from build123d import *

# Parameters (mm, degrees)
SKETCH1_W                    = 220
SKETCH1_H                    = 120
BOSS_EXTRUDE1_DEPTH          = 10
CUT_EXTRUDE1_REACH           = 127.698
SKETCH2_W                    = 20.632503002
SKETCH2_H                    = 54.730004003
F_12_5_12_5_DIAMETER_HOLE1_D = 12.5
F_10_0_10_DIAMETER_HOLE1_D   = 10
F_5_0MM_DOWEL_HOLE1_D        = 5
CUT_EXTRUDE2_REACH           = 127.698
SKETCH12_R                   = 4
SKETCH12_W                   = 81.05559148
SKETCH12_H                   = 15.93559148
SKETCH12_W_2                 = 21.30559148
SKETCH12_H_2                 = 20.21559148
SKETCH12_W_3                 = 21.55559148
DRAFT1_ANGLE                 = -1
F_8_0MM_DOWEL_HOLE1_D        = 8
M8_CLEARANCE_HOLE1_D         = 8.4


with BuildPart() as part:
    # Sketch1 → Boss-Extrude1 (new body)
    with BuildSketch(Plane(origin=(0, 0, 0), x_dir=(1, 0, 0), z_dir=(0, 1, 0))):
        Rectangle(SKETCH1_W, SKETCH1_H)
    extrude(amount=-BOSS_EXTRUDE1_DEPTH)

    # Sketch2 → Cut-Extrude1 (cut, up to next)
    with BuildSketch(Plane(origin=(0, 0, 0), x_dir=(1, 0, 0), z_dir=(0, 1, 0)), mode=Mode.PRIVATE) as cut_extrude1_sk1:
        with Locations((-99.683748499, 32.634997999)):
            Rectangle(SKETCH2_W, SKETCH2_H)
    cut_extrude1_tool1 = extrude(cut_extrude1_sk1.sketch, amount=-CUT_EXTRUDE1_REACH, mode=Mode.PRIVATE) & part.part
    add(cut_extrude1_tool1.solids().sort_by_distance((-99.683748, 0, -32.634998))[0], mode=Mode.SUBTRACT)

    # Ø12.5 (12.5) Diameter Hole1 (through all)
    with Locations(Plane(origin=(0, -10, 0), x_dir=(-1, 0, 0), z_dir=(0, -1, 0))):
        with Locations((-98, 30), (-78, 30), (70, 30), (-98, -30.5), (-78, -30.5), (70, -27.22)):
            Hole(F_12_5_12_5_DIAMETER_HOLE1_D / 2)

    # Ø10.0 (10) Diameter Hole1 (through all)
    with Locations(Plane(origin=(0, -10, 0), x_dir=(-1, 0, 0), z_dir=(0, -1, 0))):
        with Locations((-60, -7.72), (-35, -7.72), (-10, -7.72), (15, -7.72)):
            Hole(F_10_0_10_DIAMETER_HOLE1_D / 2)

    # Ø5.0mm Dowel Hole1 (through all)
    with Locations(Plane(origin=(0, -10, 0), x_dir=(-1, 0, 0), z_dir=(0, -1, 0))):
        with Locations((30, -43.22), (55, -31.22)):
            Hole(F_5_0MM_DOWEL_HOLE1_D / 2)

    # Sketch12 → Cut-Extrude2 (cut, up to next)
    with BuildSketch(Plane.XZ.offset(10), mode=Mode.PRIVATE) as cut_extrude2_sk1:
        with Locations(Location((-90, 14.72, 0), (0, 0, 270))):
            Circle(SKETCH12_R)
    cut_extrude2_tool1 = extrude(cut_extrude2_sk1.sketch, amount=-CUT_EXTRUDE2_REACH, mode=Mode.PRIVATE) & part.part
    # Sketch12 → Cut-Extrude2 (cut, up to next)
    with BuildSketch(Plane.XZ.offset(10), mode=Mode.PRIVATE) as cut_extrude2_sk2:
        with Locations(Location((-70, -0.28, 0), (0, 0, 270))):
            Circle(SKETCH12_R)
    cut_extrude2_tool2 = extrude(cut_extrude2_sk2.sketch, amount=-CUT_EXTRUDE2_REACH, mode=Mode.PRIVATE) & part.part
    # Sketch12 → Cut-Extrude2 (cut, up to next)
    with BuildSketch(Plane.XZ.offset(10), mode=Mode.PRIVATE) as cut_extrude2_sk3:
        with Locations(Location((-50, 14.72, 0), (0, 0, 270))):
            Circle(SKETCH12_R)
    cut_extrude2_tool3 = extrude(cut_extrude2_sk3.sketch, amount=-CUT_EXTRUDE2_REACH, mode=Mode.PRIVATE) & part.part
    # Sketch12 → Cut-Extrude2 (cut, up to next)
    with BuildSketch(Plane.XZ.offset(10), mode=Mode.PRIVATE) as cut_extrude2_sk4:
        with Locations(Location((-30, -0.28, 0), (0, 0, 270))):
            Circle(SKETCH12_R)
    cut_extrude2_tool4 = extrude(cut_extrude2_sk4.sketch, amount=-CUT_EXTRUDE2_REACH, mode=Mode.PRIVATE) & part.part
    # Sketch12 → Cut-Extrude2 (cut, up to next)
    with BuildSketch(Plane.XZ.offset(10), mode=Mode.PRIVATE) as cut_extrude2_sk5:
        with Locations((20, 32.16)):
            Rectangle(SKETCH12_W, SKETCH12_H)
    cut_extrude2_tool5 = extrude(cut_extrude2_sk5.sketch, amount=-CUT_EXTRUDE2_REACH, mode=Mode.PRIVATE) & part.part
    # Sketch12 → Cut-Extrude2 (cut, up to next)
    with BuildSketch(Plane.XZ.offset(10), mode=Mode.PRIVATE) as cut_extrude2_sk6:
        with Locations((-9.875, -18.86)):
            Rectangle(SKETCH12_W_2, SKETCH12_H_2)
    cut_extrude2_tool6 = extrude(cut_extrude2_sk6.sketch, amount=-CUT_EXTRUDE2_REACH, mode=Mode.PRIVATE) & part.part
    # Sketch12 → Cut-Extrude2 (cut, up to next)
    with BuildSketch(Plane.XZ.offset(10), mode=Mode.PRIVATE) as cut_extrude2_sk7:
        with Locations((30, -18.86)):
            Rectangle(SKETCH12_W_3, SKETCH12_H_2)
    cut_extrude2_tool7 = extrude(cut_extrude2_sk7.sketch, amount=-CUT_EXTRUDE2_REACH, mode=Mode.PRIVATE) & part.part
    add(cut_extrude2_tool1.solids().sort_by_distance((-90, -10, 14.72))[0], mode=Mode.SUBTRACT)
    add(cut_extrude2_tool2.solids().sort_by_distance((-70, -10, -0.28))[0], mode=Mode.SUBTRACT)
    add(cut_extrude2_tool3.solids().sort_by_distance((-50, -10, 14.72))[0], mode=Mode.SUBTRACT)
    add(cut_extrude2_tool4.solids().sort_by_distance((-30, -10, -0.28))[0], mode=Mode.SUBTRACT)
    add(cut_extrude2_tool5.solids().sort_by_distance((20, -10, 32.16))[0], mode=Mode.SUBTRACT)
    add(cut_extrude2_tool6.solids().sort_by_distance((-9.875, -10, -18.86))[0], mode=Mode.SUBTRACT)
    add(cut_extrude2_tool7.solids().sort_by_distance((30, -10, -18.86))[0], mode=Mode.SUBTRACT)

    # Draft1
    draft1_faces = [part.faces().sort_by_distance(p)[0] for p in [
        (60.52779574, -5, 32.16),
        (20, -5, 40.12779574),
        (-20.52779574, -5, 32.16),
        (20, -5, 24.19220426),
        (-9.875, -5, -8.75220426),
        (30, -5, -8.75220426),
        (40.77779574, -5, -18.86),
        (0.77779574, -5, -18.86),
        (-20.52779574, -5, -18.86),
        (19.22220426, -5, -18.86),
        (30, -5, -28.96779574),
        (-9.875, -5, -28.96779574),
        (-50, -5, 18.72),
        (-30, -5, 3.72),
        (-70, -5, 3.72),
        (-90, -5, 18.72),
    ]]
    draft(draft1_faces, Plane.ZX, DRAFT1_ANGLE)

    # Ø8.0mm Dowel Hole1 (through all)
    with Locations(Plane(origin=(0, -10, 0), x_dir=(-1, 0, 0), z_dir=(0, -1, 0))):
        with Locations((76.6, -48), (-79.6, 48)):
            Hole(F_8_0MM_DOWEL_HOLE1_D / 2)

    # M8 Clearance Hole1 (through all)
    with Locations(Plane(origin=(0, 0, 0), x_dir=(1, 0, 0), z_dir=(0, 1, 0))):
        with Locations((-95, -48), (98, -48), (98, 48), (-77.367496998, 48)):
            Hole(M8_CLEARANCE_HOLE1_D / 2)


solid = part.part
CAD build for the part. Positions are in the model's coordinates, mm. A direction names the side the tool comes from. Coordinates: 2 decimals unless noted, no trailing zeros. Loops run counter-clockwise (first coordinate to the right, second up) from the corner with the lowest first, then second, coordinate; pieces in that order, holes last. Notation, with made-up numbers: (15.5, 82) - (51.5, 82) arc R22 cw to (51.5, 91) - close; hole circle Ø10 at (-18, -21.5). An arc over 180 degrees is marked (long way). Write item = value, one per line. Start each with the question number.
Q1. Cut at A-A, the plane z = 48. List the corners of the cut face in (x, y), then the cut area to 3 significant figures.
Q2. Pull direction Z, two halves, no side cores. Call faces 1 (the flat face through (-2, -5, 60)), 2 (the conical face through (-93.627, -5.07, 12.833)), 3 (the flat face through (-2, 0, -1)): pulls with the +Z half, pulls with the -Z half, needs draft (parallel to the pull), parting line crosses it, or undercut.
Q3. Cut at C-C, the plane x = -15. List the corners of the cut face in (y, z).
Q4. Cut at D-D, the plane z = -0.28. Give the number of separate pieces and of enclosed holes in the cut face, then the cut area to 3 significant figures.
Q5. Cut at B-B, the plane x = 98. List the corners of the cut face in (y, z).
Q6. Flat gauge pin, fed straight in: pin 1 Ø10 at (x, z) = (-70, 27.22) entering from -Y. Where does the tip first touch, or does it go through?
Q7. Which spindle directions (+Z, -Z, +X, -X, +Y, -Y) get a long thin tool onto all of the face, cutting with end or side? Do faces 4 (the flat face through (-100, -5, -5.27)), 5 (the cylindrical face through (-97.26, -5.07, 44.46)). Say none if no direction does.
Q8. Drill centre lines: L1, parallel to X at y = -8.5, z = -9.5; L2, parallel to X at y = -1, z = -10.5; L3, parallel to Z at x = 98, y = -6.25. Where is each one in solid material? Low to high.
Computed:
q1.outline = (-110, -10) - (-99.2, -10) - (-99.2, 0) - (-110, 0) - close; (-90.8, -10) - (-80.6, -10) - (-80.6, 0) - (-90.8, 0) - close; (-72.6, -10) - (93.8, -10) - (93.8, 0) - (-72.6, 0) - close; (102.2, -10) - (110, -10) - (110, 0) - (102.2, 0) - close
q1.area = 1,950 mm²
q2.face_1 = pulls with the +Z half
q2.face_2 = undercut
q2.face_3 = needs draft
q3.outline = (-10, -60) - (0, -60) - (0, -28.97) - (-10, -29.14) - close; (-10, -8.58) - (0, -8.75) - (0, 2.72) - (-10, 2.72) - close; (-10, 12.72) - (0, 12.72) - (0, 24.19) - (-10, 24.02) - close; (-10, 40.3) - (0, 40.13) - (0, 60) - (-10, 60) - close
q4.separate_pieces = 3
q4.enclosed_holes = 0
q4.area = 2,040 mm²
q5.outline = (-10, -60) - (0, -60) - (0, -52.2) - (-10, -52.2) - close; (-10, -43.8) - (0, -43.8) - (0, -36.25) - (-10, -36.25) - close; (-10, -23.75) - (0, -23.75) - (0, 24.25) - (-10, 24.25) - close; (-10, 36.75) - (0, 36.75) - (0, 43.8) - (-10, 43.8) - close; (-10, 52.2) - (0, 52.2) - (0, 60) - (-10, 60) - close
q6.pin_1 = through
q7.face_4 = -Z, -X, +Y, -Y
q7.face_5 = +Y, -Y
q8.L1 = -89.37 to -20.68, 0.93 to 19.07, 40.93 to 110
q8.L2 = -89.37 to -20.55, 0.8 to 19.2, 40.8 to 110
q8.L3 = -60 to -52.2, -43.8 to -36.25, -23.75 to 24.25, 36.75 to 43.8, 52.2 to 60
